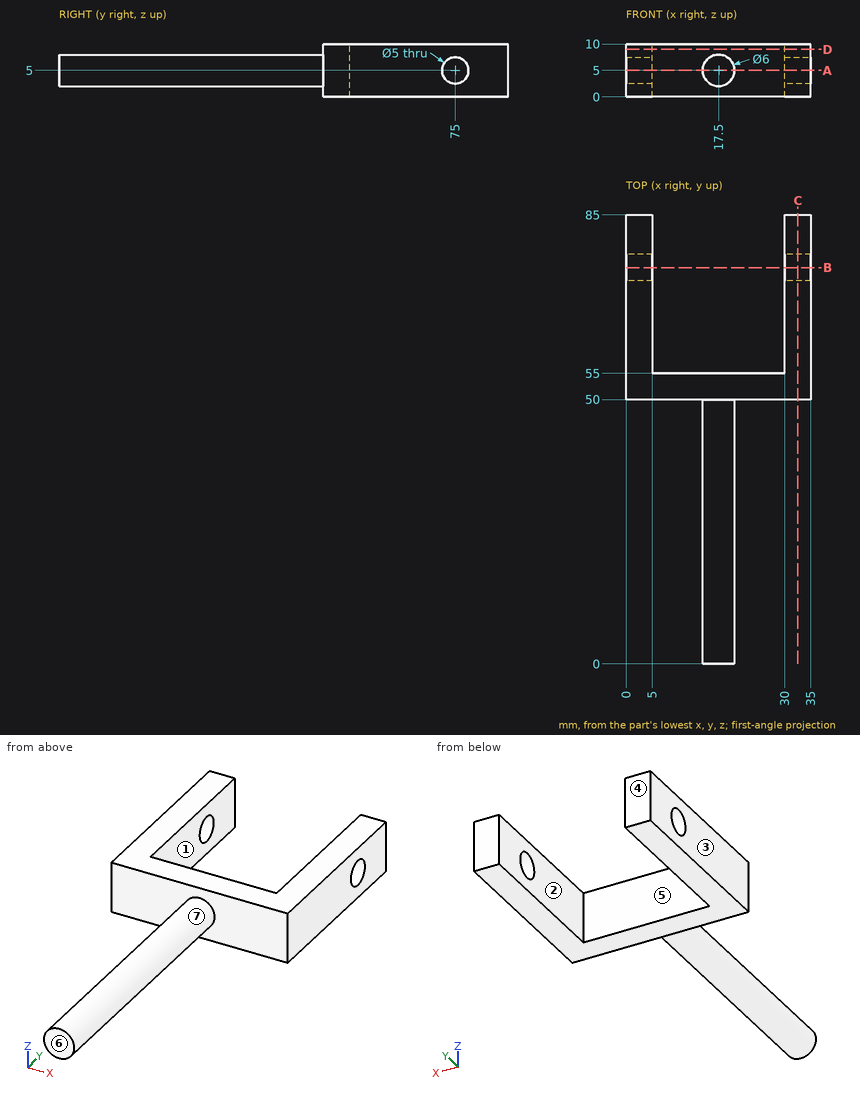
Study the drawing (mm; zero at the part's minimum x, y, z) and answer. A direction names the side the tool comes from. Round coordinates to 2 decimals unless told otherwise and drop trailing zeros. Loops run counter-clockwise (first coordinate to the right, second up) from the corner with the lowest first, then second, coordinate; pieces in that order, holes last. Notation, with made-up numbers: (3, 65) - (32, 65) arc R23 ccw to (32, 100) - close; hole circle Ø7 at (-29.75, -9.75). An arc over 180 degrees is marked (long way). Use one line per item in the form item = value. Start each with the question number.
1. Given pin 1 Ø2 at (y, z) = (39.5, 7) entering from +X; pin 2 Ø2 at (x, z) = (6, 5.5) entering from -Y; pin 3 Ø1 at (x, z) = (7.5, 4) entering from +Y, each flat-ended and moving along its own axis, determine where each tip first touches the part or whether it passes through.
2. The part is cut by section B-B on y = 75. Determine the outline of the cut face in (x, z).
3. The part is cut by section C-C on x = 32.5. Determine the outline of the cut face in (y, z).
4. For a pull along X with two mould halves and no side action, classify the marked faces 1, 2, 3 and 4 as pulls with the +X half, pulls with the -X half, needs draft (parallel to the pull), parting line crosses it, or undercut.
5. Consider line 1 (Z direction, x = 2.6, y = 75); line 2 (X direction, y = 62.5, z = 9.5); line 3 (Y direction, x = 2.25, z = 5). Determine where each line is inside the solid, lowest interval first. Write a range as [from, to].
6. The part is cut by section D-D on z = 9. Determine the outline of the cut face in (x, y), then the cut area to 3 significant figures.
7. A tool of negligible diameter and unlimited length cuts with its end or side. For the marked faces 5, 6 and 7, from which of +Z, -Z, +X, -X, +Y, -Y can it reach the whole face along a straight path? Write none if from no direction.
8. The part is cut by section A-A on z = 5. Determine the outline of the cut face in (x, y).
Geometry check:
q1.pin_1 = 20.33
q1.pin_2 = 50
q1.pin_3 = 55
q2.outline = (0, 0) - (5, 0) - (5, 2.5) - (0, 2.5) - close; (0, 7.5) - (5, 7.5) - (5, 10) - (0, 10) - close; (30, 0) - (35, 0) - (35, 2.5) - (30, 2.5) - close; (30, 7.5) - (35, 7.5) - (35, 10) - (30, 10) - close
q3.outline = (50, 0) - (85, 0) - (85, 10) - (50, 10) - close; hole circle Ø5 at (75, 5)
q4.face_1 = undercut
q4.face_2 = undercut
q4.face_3 = pulls with the -X half
q4.face_4 = needs draft
q5.line_1 = [0, 2.5], [7.5, 10]
q5.line_2 = [0, 5], [30, 35]
q5.line_3 = [50, 72.5], [77.5, 85]
q6.outline = (0, 50) - (35, 50) - (35, 85) - (30, 85) - (30, 55) - (5, 55) - (5, 85) - (0, 85) - close
q6.area = 475 mm^2
q7.face_5 = +Z, -Z, +Y
q7.face_6 = +Z, -Z, +X, -X, -Y
q7.face_7 = -Y
q8.outline = (0, 50) - (14.5, 50) - (14.5, 0) - (20.5, 0) - (20.5, 50) - (35, 50) - (35, 72.5) - (30, 72.5) - (30, 55) - (5, 55) - (5, 72.5) - (0, 72.5) - close; (0, 77.5) - (5, 77.5) - (5, 85) - (0, 85) - close; (30, 77.5) - (35, 77.5) - (35, 85) - (30, 85) - close
